The listing builds one solid part. Answer for the finished solid, in the listing's coordinates (mm). A direction names the side the tool comes from. Round coordinates to 2 decimals unless told otherwise and drop trailing zeros. Order: outer loops, then holes, each group sorted by start corner. A loop starts at its lowest first (then second) coordinate and runs counter-clockwise, first axis right, second up. Notation, with made-up numbers: M 28,24 L 65,24 A13 ccw 65,49 Z; hole C 63,63 d11. An arc over 180 degrees is marked long. Write item = value, one per line. Start each with the question number.
(1) Each of these flat-tipped pins is pushed along its axis until it touches: pin 1 (1.5 mm diameter, centred on y = 3, z = -2.5, fed in from -X); pin 2 (2 mm diameter, centred on x = -2.5, y = 4, fed in from +Z); pin 3 (4 mm diameter, centred on y = 12, z = -2.5, fed in from -X). Where does it stop, or does it pass through?
(2) For a pull along Z with two mould halves and no side action, classify faces 1 (the face through (-1.557, 24.028, -0.428)), 2 (the face through (-1, 20, 1)), 3 (the face through (-0.867, 9.614, 3.905)), 4 (the face through (-0.646, 24.028, -1.492)) as released by +Z, released by -Z, zero draft, split by the parting line, or undercut.
(3) Straight lines are drawn through the part: probe 1 along Y at (x, z) = (-2.5, 0); probe 2 along X at (y, z) = (11.5, -1); probe 3 along Z at (x, y) = (0, 21.5). For each, find the intervals that lie inside material, in ascending order. Write a range as from..to.
(4) Which of the six approach directions +Z, -Z, +X, -X, +Y, -Y give full straight-line access (tool end or side, diameter ignored) to faces 5 (the face through (0, 21, 1)), 6 (the face through (0, 26.1, 0)), 7 (the face through (1.37, 24.03, 0.85)), 8 (the face through (0.2, 24.03, 1.61)), 9 (the face through (0, 0, 0))?
(5) A cutting plane is placed at A-A, the plane y = 13. Determine the outline of the cut face in (x, z).
from build123d import *

# Parameters (mm, degrees)
CUT_EXTRUDE1_DEPTH = 4
CIRPATTERN1_COUNT  = 11


with BuildPart() as part:
    # Sketch1 → Revolve1 (revolve)
    with BuildSketch(Plane.XY):
        with BuildLine():
            Line((0, 0), (0, 26.1))
            Line((0, 26.1), (1, 26.1))
            Line((1, 26.1), (1, 26))
            Line((1, 26), (2, 26))
            Line((2, 26), (2, 22))
            Line((2, 22), (1, 22))
            Line((1, 22), (1, 20))
            Line((1, 20), (3.5, 20))
            ThreePointArc((3.5, 20), (3.853553391, 19.853553391), (4, 19.5))
            Line((4, 19.5), (4, 0))
            Line((4, 0), (0, 0))
        make_face()
    revolve(axis=Axis((0, 0, 0), (0, 1, 0)))

    # Sketch2 → Cut-Extrude1 (cut)
    with BuildSketch(Plane(origin=(0, 26, 0), x_dir=(1, 0, 0), z_dir=(0, 1, 0))):
        with BuildLine():
            ThreePointArc((-0.5, 1.936491673), (0, 2), (0.5, 1.936491673))
            ThreePointArc((0.5, 1.936491673), (0.260400333, 1.599188187), (0.095331419, 1.219801979))
            ThreePointArc((0.095331419, 1.219801979), (0, 1.15), (-0.095331419, 1.219801979))
            ThreePointArc((-0.095331419, 1.219801979), (-0.260400333, 1.599188187), (-0.5, 1.936491673))
        make_face()
    cut_extrude1 = extrude(amount=-CUT_EXTRUDE1_DEPTH, mode=Mode.SUBTRACT)

    # CirPattern1: Cut-Extrude1 ×11 about axis
    cirpattern1_axis = Axis((0, 0, 0), (0, 1, 0))
    for i in range(1, CIRPATTERN1_COUNT):
        add(cut_extrude1.rotate(cirpattern1_axis, i * 360 / CIRPATTERN1_COUNT), mode=Mode.SUBTRACT)


solid = part.part
Reported:
q1.pin_1 = -3.6
q1.pin_2 = 3.71
q1.pin_3 = -3.97
q2.face_1 = undercut
q2.face_2 = zero draft
q2.face_3 = split by the parting line
q2.face_4 = undercut
q3.probe_1 = 0..20
q3.probe_2 = -3.87..3.87
q3.probe_3 = -1..1
q4.face_5 = none
q4.face_6 = +Z, -Z, +X, -X, +Y
q4.face_7 = +Y
q4.face_8 = +Z, +Y
q4.face_9 = +Z, -Z, +X, -X, -Y
q5.outline = C 0,0 d8
